Source: CAD feature listing. Evaluate the final solid. Frame: model axes, mm. A direction names the side the tool comes from. Give positions to 0.01 mm unless a question says otherwise; leave off trailing zeros. Write each loop counter-clockwise with the first axis right and the second up, starting at its lowest first coordinate (ties: lowest second). Pieces come first, ordered by that corner, then holes. Notation, with made-up numbers: (-29, -11.75) -> (-20, -11.75) arc R26 ccw to (-20, 14.25) -> close; hole circle Ø4 at (70.5, 61). An arc over 180 degrees is marked (long way). Write item = value, one per line.
from build123d import *

# Parameters (mm, degrees)
F1_DEPTH = 0.5
F3_W     = 8
F3_H     = 8
F4_DEPTH = 0.5


with BuildPart() as f1:
    # F0 (on Front) → F1 (new body)
    with BuildSketch(Plane.XZ):
        Polygon((6, 0), (0, 0), (0, -8), (6, -8), (10.472136, -4), align=None)
    extrude(amount=F1_DEPTH)

    # F3 (on face) → F4 (join)
    with BuildSketch(Plane(origin=(0.160697, -0.441511, 0), x_dir=(0.939693, 0.34202, 0), z_dir=(0.34202, -0.939693, 0))):
        with Locations((-4, -4)):
            Rectangle(F3_W, F3_H)
    extrude(amount=-F4_DEPTH)


solid = f1.part
(1) First-contact query: pin 1 (2 mm diameter, centred on x = 7.5, z = -3, fed in from -Y); pin 2 (1 mm diameter, centred on x = 3.5, z = -1, fed in from +Y). Flat tips, straight axial feed; report the tip coordinate or a pass-through.
Values follow:
pin_1 = -0.5
pin_2 = 0
(2) Section query D-D (y = -1.05). Return loops of the section in (x, z), plus the area to 3 significant figures.
Values follow:
outline = (-2.97, -8) -> (-1.51, -8) -> (-1.51, 0) -> (-2.97, 0) -> close
area = 11.7 mm2
(3) Section query B-B (x = 2). Return loops of the section in (y, z), plus the area to 3 significant figures.
Values follow:
outline = (-0.5, -8) -> (0, -8) -> (0, 0) -> (-0.5, 0) -> close
area = 4.00 mm2
(4) Access query for faces 4 (the face through (4, -0.5, -4)), 5 (the face through (8.27, -0.25, -2.03)), 6 (the face through (4, 0, -4)). Directions: +Z, -Z, +X, -X, +Y, -Y. A direction counts if a zero-diameter tool reaches every point of the face in a straight line with its end or side. Return the directions, or none.
Values follow:
face_4 = +Z, -Z, +X, -Y
face_5 = +Z, +X, +Y, -Y
face_6 = +Z, -Z, +X, +Y
(5) Material intervals for line 1 (Y direction, x = 3.5, z = -3); line 2 (Y direction, x = -2.5, z = -3), sorted ascending.
Values follow:
line_1 = -0.5 to 0
line_2 = -1.41 to -0.88
(6) Pull-direction query (Z, two-part tool) for faces 1 (the face through (8.2, -0.25, -6.03)), 2 (the face through (-3.82, -1.36, -3.94)), 3 (the face through (-0.6, -0.5, 0)); classes: pulls with the +Z half, pulls with the -Z half, needs draft (parallel to the pull), parting line crosses it, or undercut.
Values follow:
face_1 = pulls with the -Z half
face_2 = needs draft
face_3 = pulls with the +Z half
